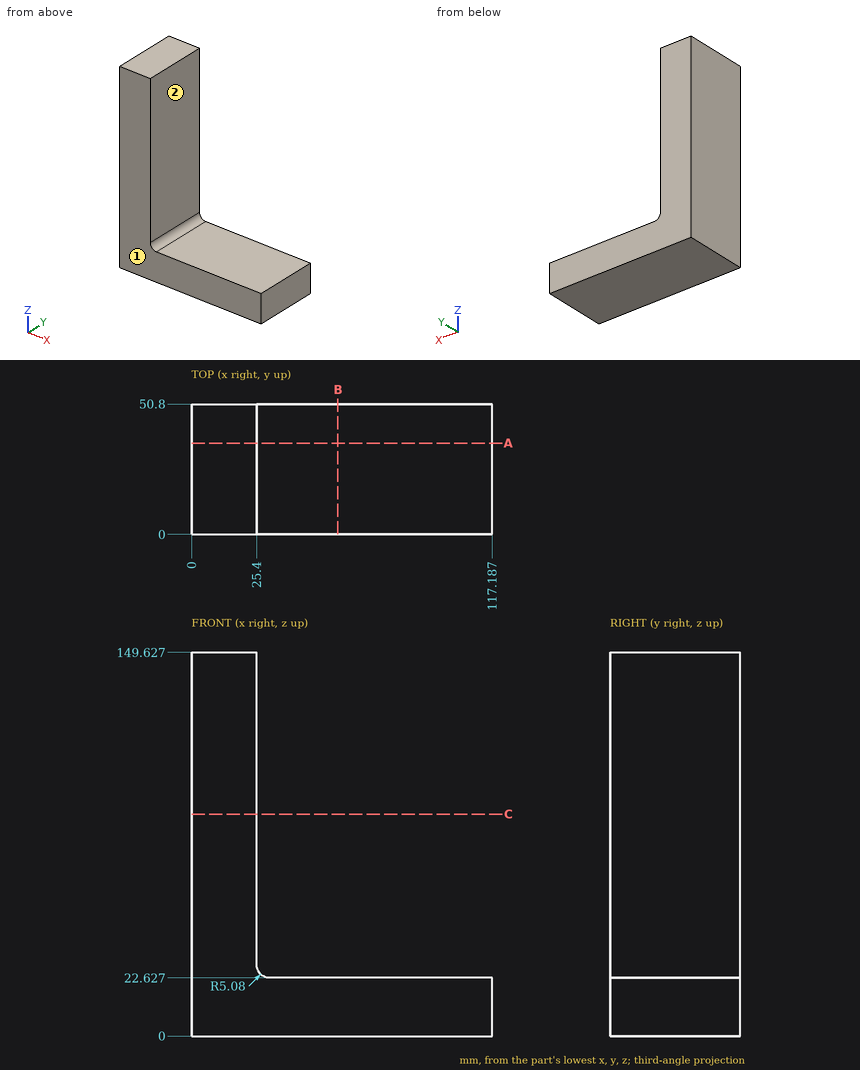
Geometry: see drawing. Coordinates: mm, zero at the bounding-box minimum. A direction names the side the tool comes from. Give positions to 0.01 mm unless a question says otherwise; leave off trailing zeros. Order: outer loops, then holes, each group sorted by start corner. A loop starts at its lowest first (then second) coordinate and runs counter-clockwise, first axis right, second up. Notation, with made-up numbers: M 82.25,-6 L 132.25,-6 A18 cw 132.25,25 Z; hole C 21,48.5 d11. An arc over 180 degrees is marked long. Answer as a JSON object with one key per item and string values.
1. Ray query, line 1 (Z direction, x = 40, y = 3.5); line 2 (X direction, y = 18, z = 50); line 3 (Z direction, x = 26, y = 28). Return the intervals inside material, ascending. Write a range as [from, to].
Result sheet:
{"line 1": "[0, 22.63]", "line 2": "[0, 25.4]", "line 3": "[0, 25.31]"}
2. Cut plane C-C, the plane z = 86.5. Output: boundary loops of the cut face in (x, y), and give its area (3 significant figures).
Result sheet:
{"outline": "M 0,0 L 25.4,0 L 25.4,50.8 L 0,50.8 Z", "area": "1,290 mm²"}
3. Cut plane B-B, the plane x = 57. Output: boundary loops of the cut face in (y, z).
Result sheet:
{"outline": "M 0,0 L 50.8,0 L 50.8,22.63 L 0,22.63 Z"}
4. First-contact query: P1, Ø15, axis at y = 33.5, z = 78, coming from the +X side. Flat tip, straight axial feed; report the tip coordinate or a pass-through.
Result sheet:
{"P1": "x = 25.4"}
5. Cut plane A-A, the plane y = 35.5. Output: boundary loops of the cut face in (x, z), and give its area (3 significant figures).
Result sheet:
{"outline": "M 0,0 L 117.19,0 L 117.19,22.63 L 30.48,22.63 A5.08 cw 25.4,27.71 L 25.4,149.63 L 0,149.63 Z", "area": "5,880 mm²"}
6. Reachability of the marked faces 1 and 2 from +Z, -Z, +X, -X, +Y, -Y: full face, straight path, thin tool, end or side. Return the list, or none.
Result sheet:
{"face 1": "+Z, -Z, +X, -X, -Y", "face 2": "+Z, +X, +Y, -Y"}
